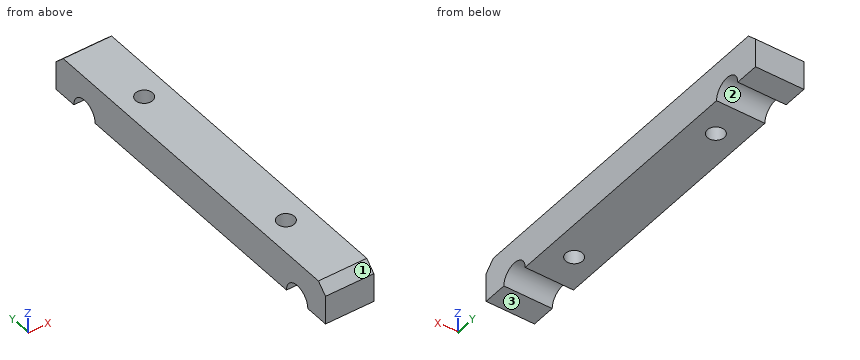
Autodesk Inventor part; units mm, degrees
ref_plane "YZ Plane" through (0, 0, 0) normal (1, 0, 0) x (0, 1, 0)
ref_plane "XZ Plane" through (0, 0, 0) normal (0, 1, 0) x (-1, 0, 0)
ref_plane "XY Plane" through (0, 0, 0) normal (0, 0, 1) x (1, 0, 0)
sketch "Szkic1" plane through (0, 0, 0) normal (1, 0, 0) x (0, 1, 0)
  circle A0 centre (0, 0) radius 3 construction
  circle A1 centre (60, 0) radius 3 construction
  arc A2 (63, 0) -> (57, 0) centre (60, 0) ccw
  arc A3 (3, 0) -> (-3, 0) centre (0, 0) ccw
  line L0 (68, 0) -> (68, 8)
  line L1 (68, 8) -> (-8, 8)
  line L2 (-8, 8) -> (-8, 0)
  line L3 (63, 0) -> (68, 0)
  line L4 (-8, 0) -> (-3, 0)
  line L5 (3, 0) -> (57, 0)
  point P0 (-5.5, 0)
  dimension "d0" = 6
  dimension "d1" = 6
  dimension "d2" = 60
  dimension "d3" = 6
  dimension "d4" = 5
  dimension "d5" = 8
extrude "Wyciągnięcie proste1" add sketch "Szkic1" along normal blind 10
sketch "Szkic2" plane through (0, 3, 0) normal (0, 0, -1) x (-1, 0, 0)
  line L0 (0, 65) -> (-10, 65) construction
  line L1 (-5, 65) -> (-5, -11.1641) construction
  line L2 (-10, 65) -> (-10, -11) construction
  line L3 (-10, 27) -> (0, 27) construction
  line L4 (0, 65) -> (0, -11) construction
  circle A0 centre (-5, 47) radius 1.75
  circle A1 centre (-5, 7) radius 1.75
  circle A2 centre (-5, 37) radius 1.75
  circle A3 centre (-5, 17) radius 1.75
  point P0 (0, -3)
  dimension "d8" = 3.5
  dimension "d9" = 20
  dimension "d15" = 3.5
  dimension "d16" = 10
extrude "Wyciągnięcie proste2" cut sketch "Szkic2" against normal up to next contours A0 | A1
chamfer "Faza1" distance 2 angle 45 2 edges at (5, 68, 8) (5, -8, 8)
ref_plane "Płaszczyzna konstrukcyjna1" through (5, 68, 6) normal (0, 1, 0) x (1, 0, 0)
sketch "Szkic3" plane through (5, 68, 6) normal (0, 1, 0) x (1, 0, 0)
  point P0 (-5, 6)
sketch "Szkic4" plane through (5, 68, 6) normal (0, 1, 0) x (1, 0, 0)
  line L0 (29.238, 4.1877) -> (10.4797, -9.1212)
  line L1 (11.1628, -10.084) -> (10.4797, -9.1212)
  line L2 (13.5481, -13.4459) -> (11.1628, -10.084)
  line L3 (29.9211, 3.2248) -> (29.238, 4.1877)
  line L4 (29.9211, 3.2248) -> (32.3064, -0.1371)
  point P0 (-5, 6)
ref_plane "Płaszczyzna konstrukcyjna2" through (17.8649, 60.2933, 18.4831) normal (-0.5693, 0.1792, -0.8024) x (0.1037, 0.9838, 0.1462)
ref_plane "Płaszczyzna konstrukcyjna3" through (26.0515, 48.9795, 10.1477) normal (-0.5693, 0.1792, -0.8024) x (0.8156, 0, -0.5786)
sketch "Szkic5" plane through (26.0515, 48.9795, 10.1477) normal (-0.5693, 0.1792, -0.8024) x (0.8156, 0, -0.5786)
  line L0 (11.5, -11.5) -> (11.5, 11.5) construction
  line L1 (11.5, 11.5) -> (-11.5, 11.5) construction
  line L2 (-11.5, 11.5) -> (-11.5, -11.5) construction
  line L3 (-11.5, -11.5) -> (11.5, -11.5) construction
  line L4 (-11.5, 11.5) -> (18.547, 11.5)
  line L5 (18.547, 11.5) -> (18.547, -17.121)
  line L6 (18.547, -17.121) -> (-11.5, -17.121)
  line L7 (-11.5, -17.121) -> (-11.5, 11.5)
  circle A0 centre (14.589, 7.796) radius 1.45
  line L8 (18.547, -17.121) -> (-11.5, 11.5) construction
  circle A1 centre (-6.5329, -14.3782) radius 1.45
  point P0 (-15.3751, 52.3715)
  dimension "d17" = 30.047
  dimension "d18" = 2.9
  dimension "d19" = 3.704
  dimension "d20" = 3.958
  dimension "d21" = 28.621
extrude "Wyciągnięcie proste3" [suppressed]
sketch "Szkic6" plane through (18.5909, 67.18, 19.5063) normal (0.1037, 0.9838, 0.1462) x (0.8156, 0, -0.5786)
  line L0 (0, 0) -> (30, 0)
  line L1 (30, 0) -> (30, 4)
  line L2 (0, 4) -> (30, 4)
  line L3 (0, 0) -> (0, 4)
  line L4 (2, 7) -> (26.5831, 7)
  line L5 (26.5831, 7) -> (26.5831, 10)
  line L6 (26.5831, 10) -> (0, 10)
  line L7 (0, 10) -> (0, 4)
  arc A0 (2, 7) -> (2, 4) centre (2, 5.5) ccw
  point P0 (-3.8751, 14.1945)
  dimension "d24" = 3
  dimension "d25" = 2.042
  dimension "d26" = 3.062
extrude "Wyciągnięcie proste4" [suppressed]
sketch "Szkic7" plane through (34.5787, 68.9722, -3.8997) normal (-0.5693, 0.1792, -0.8024) x (-0.8156, 0, 0.5786)
  line L0 (26.5831, -27.9454) -> (26.3218, -30)
  line L1 (26.5831, 0) -> (26.5831, -27.9454)
  line L2 (0, 0) -> (26.5831, 0)
  line L3 (0, 0) -> (0, -30)
  line L4 (0, -30) -> (26.3218, -30)
  line L5 (0, -20) -> (0, -10)
  line L6 (0, 0) -> (0, -30)
  line L7 (26.5831, 0) -> (26.5831, -26.8739)
  circle A0 centre (4, -15) radius 1.45
  line L8 (26.5831, 0) -> (26.5831, -30)
  line L9 (26.5831, -30) -> (21.5831, -30)
  line L10 (-3.4169, -30) -> (24.5831, -30)
  line L11 (21.5831, -30) -> (0, -20)
  line L12 (0, -10) -> (21.5831, 0)
  line L13 (26.5831, 0) -> (21.5831, 0)
  line L14 (21.5831, -30) -> (26.5831, -30)
  point P0 (30.4582, -70.8715)
  point P1 (0, -15)
  point P2 (0, -10)
  point P3 (21.5831, -30)
  dimension "d29" = 11.638
  dimension "d32" = 2.9
  dimension "d33" = 6.646
  dimension "d34" = 3.439
extrude "Wyciągnięcie proste5" [suppressed]
sketch "Szkic11" plane through (10, 0, 0) normal (1, 0, 0) x (0, 0, -1)
  line L0 (6.8231, 49.296) -> (-4.2042, 39.4579)
  line L1 (-4.2042, 39.4579) -> (-6.9463, 39.4579)
  line L2 (-7.3978, 41.4793) -> (-6.9463, 39.4579)
  line L3 (-11.4825, 68.9722) -> (-7.3978, 41.4793)
  line L4 (-8.5893, 68.9722) -> (-11.4825, 68.9722)
  line L5 (-8.5893, 68.9722) -> (5.3614, 59.1341)
  line L6 (5.3614, 59.1341) -> (6.8231, 49.296)
  ellipse E0 centre (3.7776, 54.2151) end of major axis (4.0937, 52.7999) minor radius 0.8255
  line L7 (0, 3) -> (0, 57)
  line L8 (-8, 66) -> (-8, -6)
  line L9 (0, 43.2088) -> (0, 62.915)
  line L10 (0, 62.915) -> (-6.5007, 67.4993)
  line L11 (-6.5007, 67.4993) -> (-8, 66)
  line L12 (-8, 66) -> (-8, 45.5327)
  point P0 (0, 0)
  point P1 (0, 0)
  point P2 (0, 0)
  point P3 (0, 0)
  point P4 (0, 0)
extrude "Wyciągnięcie proste8" [suppressed]
sketch "Szkic8" plane through (10, 0, 0) normal (1, 0, 0) x (0, 0, -1)
  line L0 (-2.1469, 67.18) -> (2.2382, 37.6657)
  line L1 (2.2382, 37.6657) -> (5.4477, 38.3826)
  line L2 (1.0626, 67.8969) -> (5.4477, 38.3826)
  line L3 (-2.1469, 67.18) -> (1.0626, 67.8969)
  line L4 (1, 2.8284) -> (1, 57.1716)
  line L5 (5.3614, 59.1341) -> (6.8231, 49.296)
  arc A0 (0, 63) -> (0, 57) centre (0, 60) ccw
  line L6 (9.8159, 60) -> (9.8159, 68.4413)
  line L7 (9.8159, 68.4413) -> (-3.5, 68.4413)
  line L8 (-3.5, 68.4413) -> (-3.5, 60)
  line L9 (0, 56.5) -> (9.8159, 56.5)
  line L10 (9.8159, 56.5) -> (9.8159, 60)
  arc A1 (-3.5, 60) -> (0, 56.5) centre (0, 60) ccw
  point P0 (0, 0)
  dimension "d42" = 3.5
extrude "Wyciągnięcie proste6" [suppressed]
sketch "Szkic12" plane through (17.091, 68.1657, 13.9359) normal (0.1037, 0.9838, 0.1462) x (0.8156, 0, -0.5786)
  line L0 (20.9791, -1.5) -> (18.9515, -1.5)
  line L1 (26.5257, -5.5) -> (20.9791, -1.5)
  line L2 (24.6821, -5.5) -> (26.5257, -5.5)
  line L3 (18.9515, -1.5) -> (24.6821, -5.5)
  line L4 (28, -5.5) -> (-2, -5.5)
  line L5 (18.9515, -1.5) -> (28, -1.5)
  line L6 (28, -1.5) -> (28, -5.5)
  line L7 (28, -5.5) -> (18.9515, -5.5)
  line L8 (18.9515, -5.5) -> (18.9515, -1.5)
  point P0 (-5.8751, 8.6945)
  point P1 (18.9515, -5.5)
extrude "Wyciągnięcie proste9" [suppressed]
sketch "Szkic13" plane through (0, 0, 0) normal (-1, 0, 0) x (0, 0, 1)
  line L0 (6.5007, 67.4993) -> (8, 66)
  line L1 (8, 66) -> (8, 45.5327)
  line L2 (11.4825, 68.9722) -> (8, 45.5327)
  line L3 (8.5893, 68.9722) -> (11.4825, 68.9722)
  line L4 (8.5893, 68.9722) -> (6.5007, 67.4993)
  line L5 (63.0199, 65.5599) -> (-3.0201, 65.5599)
  line L6 (15.1212, 37.6657) -> (19.5063, 67.18)
  line L7 (19.5063, 67.18) -> (11.4825, 68.9722)
  line L8 (11.4825, 68.9722) -> (8, 45.5327)
  line L9 (8, 45.5327) -> (7.3978, 41.4793)
  line L10 (7.3978, 39.3909) -> (7.3978, 41.4793)
  line L11 (15.1212, 37.6657) -> (7.3978, 39.3909)
  line L12 (8, -6) -> (6, -8)
  line L13 (8, 66) -> (8, -6)
  line L14 (6, 68) -> (8, 66)
  line L15 (0, 68) -> (6, 68)
  line L16 (0, 63) -> (0, 68)
  arc A0 (0, 57) -> (0, 63) centre (0, 60) ccw
  line L17 (0, 3) -> (0, 57)
  arc A1 (0, -3) -> (0, 3) centre (0, 0) ccw
  line L18 (0, -8) -> (0, -3)
  line L19 (6, -8) -> (0, -8)
  line L20 (8, 66) -> (8, -6)
  line L21 (8, 39.2563) -> (0, 39.2563)
  line L22 (0, 3) -> (0, 57)
  point P0 (8, 39.2563)
extrude "Wyciągnięcie proste10" [suppressed]
sketch "Szkic14" plane through (10.4273, 45.5327, 8) normal (0.8156, 0, -0.5786) x (-0.5786, 0, -0.8156)
  point P0 (12.5583, -45.5327)
sketch "Szkic15" plane through (10.4273, 45.5327, 8) normal (0.8156, 0, -0.5786) x (-0.5786, 0, -0.8156)
  line L0 (-4.27, 23.4395) -> (0, 0)
  line L1 (0, 20.4673) -> (0, 0)
  line L2 (1.8383, 21.9666) -> (0, 20.4673)
  line L3 (1.8383, 21.9666) -> (-0.7226, 23.4395)
  line L4 (-0.7226, 23.4395) -> (-4.27, 23.4395)
  point P0 (12.5583, -45.5327)
sketch "Szkic16" plane through (0, 68, 0) normal (0, 1, 0) x (1, 0, 0)
  line L0 (0, 0) -> (43.9824, 0)
  line L1 (43.9824, 0) -> (43.9824, -26.4065)
  line L2 (43.9824, -26.4065) -> (0, -26.4065)
  line L3 (0, -26.4065) -> (0, 0)
extrude "Wyciągnięcie proste11" [suppressed]
sketch "Szkic17" plane through (0, 67, 0) normal (0, 1, 0) x (1, 0, 0)
  point P0 (0, 0)
sketch "Szkic18" plane through (0, 67, 0) normal (0, 1, 0) x (1, 0, 0)
  line L0 (20.2969, -5.7927) -> (21.0993, -8.9622)
  line L1 (20.2969, -5.7927) -> (11.6216, -12.236)
  line L2 (11.6216, -12.236) -> (8.0042, -6.3815)
  line L3 (8.0042, -6.3815) -> (20.2969, -5.7927)
  point P0 (0, 0)
extrude "Wyciągnięcie proste12" [suppressed]
sketch "Szkic19" plane through (0, 67, 0) normal (0, 1, 0) x (1, 0, 0)
  point P0 (0, 0)
properties part number "6_2xclamp_main"
Work out the finished part from the listing and answer in its coordinate system (mm). Face numbers are marked on the shaded views. Coordinates: 2 decimals unless noted, no trailing zeros. Write each loop counter-clockwise with the first axis right and the second up, starting at its lowest first coordinate (ties: lowest second). Pieces come first, ordered by that corner, then holes. Notation, with made-up numbers: M 61.5,-14.5 L 74.5,-14.5 A10 ccw 74.5,-8.5 Z; hole C 30.25,59 d6. An arc over 180 degrees is marked long. Use one line per item in the form item = value. Start each with the question number.
1. Straight lines are drawn through the part: probe 1 along Y at (x, z) = (5, 2.75); probe 2 along Y at (x, z) = (5.5, 3.5); probe 3 along Y at (x, z) = (4.5, 2.25). For each, find the intervals that lie inside material, in ascending order. Write a range as from..to.
2. The part is cut by section C-C (x = 5). Give the vertices of the cut face in (y, z).
3. The part is cut by section B-B (y = 10). Give the vertices of the cut face in (x, z).
4. The part is cut by section A-A (z = 0.75). Give the vertices of the cut face in (x, y), plus the area to 3 significant figures.
5. Each of these flat-tipped pins is pushed along its axis until it touches: P1, Ø2, axis at x = 8.5, y = 16.5, coming from the -Z side; P2, Ø2, axis at x = 5, y = 10, coming from the +Z side. Where does it stop, or does it pass through?
6. The mould has two halves that part along Y. Classify the marked faces 1, 2 and 3: released by +Y, released by -Y, zero draft, split by the parting line, or undercut.
7. The part is cut by section D-D (z = 4.25). Give the vertices of the cut face in (x, y).
Evaluation:
q1.probe_1 = -8..-1.2, 1.2..8.25, 11.75..48.25, 51.75..58.8, 61.2..68
q1.probe_2 = -8..8.32, 11.68..48.32, 51.68..68
q1.probe_3 = -8..-1.98, 1.98..8.32, 11.68..48.32, 51.68..58.02, 61.98..68
q2.outline = M -8,0 L -3,0 A3 cw 3,0 L 8.25,0 L 8.25,8 L -6,8 L -8,6 Z; M 11.75,0 L 48.25,0 L 48.25,8 L 11.75,8 Z; M 51.75,0 L 57,0 A3 cw 63,0 L 68,0 L 68,6 L 66,8 L 51.75,8 Z
q3.outline = M 0,0 L 3.25,0 L 3.25,8 L 0,8 Z; M 6.75,0 L 10,0 L 10,8 L 6.75,8 Z
q4.outline = M 0,-8 L 10,-8 L 10,-2.9 L 0,-2.9 Z; M 0,2.9 L 10,2.9 L 10,57.1 L 0,57.1 Z; M 0,62.9 L 10,62.9 L 10,68 L 0,68 Z; hole C 5,10 d3.5; hole C 5,50 d3.5
q4.area = 625 mm^2
q5.P1 = 0
q5.P2 = through
q6.face_1 = released by -Y
q6.face_2 = undercut
q6.face_3 = zero draft
q7.outline = M 0,-8 L 10,-8 L 10,68 L 0,68 Z; hole C 5,10 d3.5; hole C 5,50 d3.5
